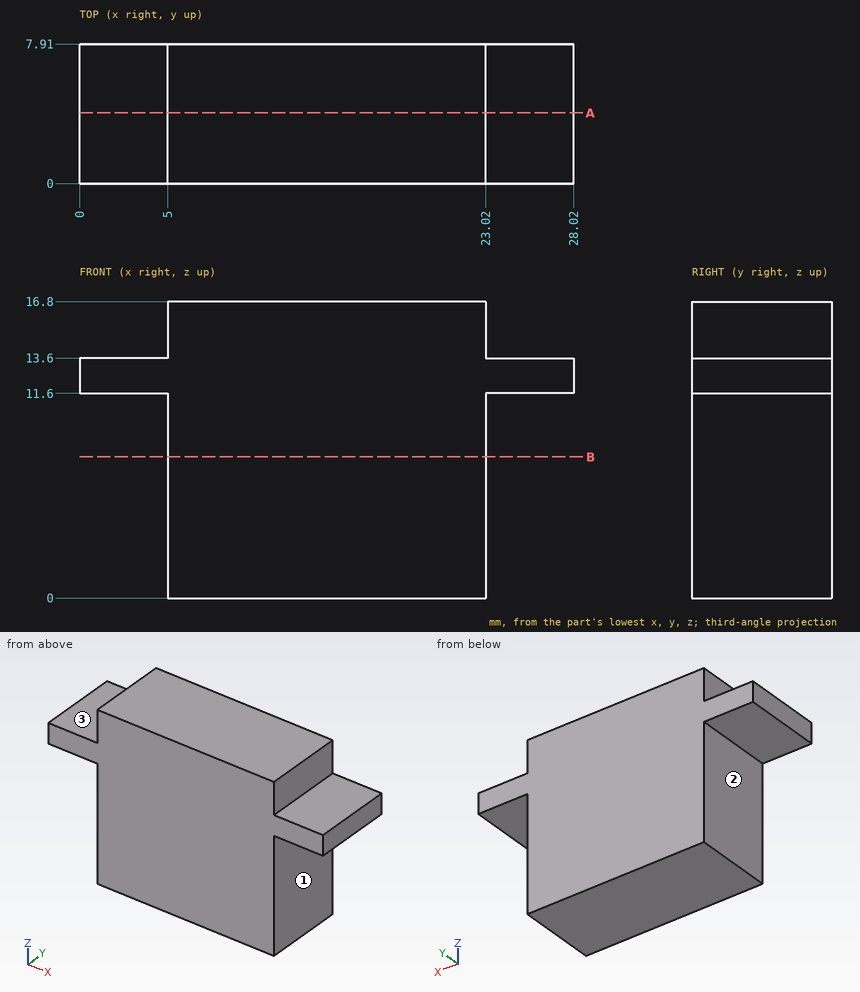
Part print with two shaded views. Sizes in mm from the minimum x, y, z corner. A direction names the side the tool comes from. Coordinates: 2 decimals unless noted, no trailing zeros. Order: outer loops, then holes, each group sorted by start corner. A loop starts at its lowest first (then second) coordinate and runs counter-clockwise, first axis right, second up. Notation, with made-up numbers: (75, 72.5) - (119, 72.5) arc R16 ccw to (119, 100.5) - close; hole circle Ø5 at (69, -17.75). An arc over 180 degrees is marked (long way). Write item = value, one per line. Start each with the question number.
1) Wall check: line 1 along X through (y, z) = (2, 14.5); line 2 along Z through (x, y) = (1, 5.5). Give the ranges that are in metal, low to high. Write a range as from..to.
2) 3-axis set-ups, long thin cutter, end or side, ignore diameter. For the marked faces 1, 2 and 3: which of +Z, -Z, +X, -X, +Y, -Y reach the whole face in a straight line?
3) Saw through at B-B on z = 8. Write the cut outline in (x, y).
4) Flat gauge pins, fed straight in: pin 1 Ø4 at (y, z) = (2, 6.5) entering from -X; pin 2 Ø1.5 at (x, y) = (26, 2.5) entering from -Z; pin 3 Ø4 at (x, y) = (3.5, 4) entering from -Z; pin 4 Ø2.5 at (x, y) = (25.5, 5) entering from +Z. Where does each tip first touch, or does it go through?
5) Saw through at A-A on y = 4. Write the cut outline in (x, z).
From the geometry:
q1.line_1 = 5..23.02
q1.line_2 = 11.6..13.6
q2.face_1 = -Z, +X, +Y, -Y
q2.face_2 = -Z, -X, +Y, -Y
q2.face_3 = +Z, -X, +Y, -Y
q3.outline = (5, 0) - (23.02, 0) - (23.02, 7.91) - (5, 7.91) - close
q4.pin_1 = 5
q4.pin_2 = 11.6
q4.pin_3 = 0
q4.pin_4 = 13.6
q5.outline = (0, 11.6) - (5, 11.6) - (5, 0) - (23.02, 0) - (23.02, 11.6) - (28.02, 11.6) - (28.02, 13.6) - (23.02, 13.6) - (23.02, 16.8) - (5, 16.8) - (5, 13.6) - (0, 13.6) - close
